```python
from build123d import *

# Parameters (mm, degrees)
F0_W        = 7.39
F0_H        = 23.34
F0_R        = 2.4
F1_DEPTH    = 7.88
F2_T1_DEPTH = 26.405
F4_DEPTH    = 7.391
F5_R        = 3.705


# Not quite as in the source:
# - a fillet or chamfer that OpenCascade refuses, or shapes differently, is made with other operations: its cross-section is extruded or revolved along the edge and cut away or added


with BuildPart() as f1:
    # F0 (on Top) → F1 (new body)
    with BuildSketch(Plane.XY):
        with Locations((-61.1013304442, -8.6294944299)):
            Rectangle(F0_W, F0_H)
        with Locations((-61.1013304442, -8.6294944299)):
            Circle(F0_R, mode=Mode.SUBTRACT)
        with Locations((-61.1013304442, -0.6294944299)):
            Circle(F0_R, mode=Mode.SUBTRACT)
    extrude(amount=F1_DEPTH)

    # F2: fillet of radius 3.705 on 2 edges, made by hand

    # F2_s2 → F2_t1 (cut)
    with BuildSketch(Plane.XY.offset(-9.2625)):
        with BuildLine():
            ThreePointArc((-61.0913304442, 3.0405055701), (-63.7111610685, 1.9553361944), (-64.7963304442, -0.6644944299))
            Line((-64.7963304442, -0.6644944299), (-64.7963304442, 3.0405055701))
            Line((-64.7963304442, 3.0405055701), (-61.0913304442, 3.0405055701))
        make_face()
        with BuildLine():
            ThreePointArc((-61.1113304442, 3.0405055701), (-58.4914998199, 1.9553361944), (-57.4063304442, -0.6644944299))
            Line((-57.4063304442, -0.6644944299), (-57.4063304442, 3.0405055701))
            Line((-57.4063304442, 3.0405055701), (-61.1113304442, 3.0405055701))
        make_face()
    extrude(amount=F2_T1_DEPTH, mode=Mode.SUBTRACT)

    # F3 (on face) → F4 (cut, through all)
    with BuildSketch(Plane.YZ.offset(-57.4063304442)):
        with BuildLine():
            Line((-15.7294944299, 5.34), (-15.7294944299, 6.0963858653))
            ThreePointArc((-15.7294944299, 6.0963858653), (-15.747402223, 6.1534898894), (-15.7947118212, 6.1901417725))
            ThreePointArc((-15.7947118212, 6.1901417725), (-16.6294944299, 6.34), (-17.4642770386, 6.1901417725))
            ThreePointArc((-17.4642770386, 6.1901417725), (-17.5115866368, 6.1534898894), (-17.5294944299, 6.0963858653))
            Line((-17.5294944299, 6.0963858653), (-17.5294944299, 5.34))
            ThreePointArc((-17.5294944299, 5.34), (-17.6759410393, 4.9864466094), (-18.0294944299, 4.84))
            Line((-18.0294944299, 4.84), (-18.7858802952, 4.84))
            ThreePointArc((-18.7858802952, 4.84), (-18.8429843193, 4.8220922069), (-18.8796362024, 4.7747826087))
            ThreePointArc((-18.8796362024, 4.7747826087), (-18.9917328021, 4.3640635248), (-19.0294944299, 3.94))
            ThreePointArc((-19.0294944299, 3.94), (-18.9917328021, 3.5159364752), (-18.8796362024, 3.1052173913))
            ThreePointArc((-18.8796362024, 3.1052173913), (-18.8429843193, 3.0579077931), (-18.7858802952, 3.04))
            Line((-18.7858802952, 3.04), (-18.0294944299, 3.04))
            ThreePointArc((-18.0294944299, 3.04), (-17.6759410393, 2.8935533906), (-17.5294944299, 2.54))
            Line((-17.5294944299, 2.54), (-17.5294944299, 1.7836141347))
            ThreePointArc((-17.5294944299, 1.7836141347), (-17.5115866368, 1.7265101106), (-17.4642770386, 1.6898582275))
            ThreePointArc((-17.4642770386, 1.6898582275), (-16.6294944299, 1.54), (-15.7947118212, 1.6898582275))
            ThreePointArc((-15.7947118212, 1.6898582275), (-15.747402223, 1.7265101106), (-15.7294944299, 1.7836141347))
            Line((-15.7294944299, 1.7836141347), (-15.7294944299, 2.54))
            ThreePointArc((-15.7294944299, 2.54), (-15.5830478205, 2.8935533906), (-15.2294944299, 3.04))
            Line((-15.2294944299, 3.04), (-14.4731085646, 3.04))
            ThreePointArc((-14.4731085646, 3.04), (-14.4160045405, 3.0579077931), (-14.3793526574, 3.1052173913))
            ThreePointArc((-14.3793526574, 3.1052173913), (-14.2672560577, 3.5159364752), (-14.2294944299, 3.94))
            ThreePointArc((-14.2294944299, 3.94), (-14.2672560577, 4.3640635248), (-14.3793526574, 4.7747826087))
            ThreePointArc((-14.3793526574, 4.7747826087), (-14.4160045405, 4.8220922069), (-14.4731085646, 4.84))
            Line((-14.4731085646, 4.84), (-15.2294944299, 4.84))
            ThreePointArc((-15.2294944299, 4.84), (-15.5830478205, 4.9864466094), (-15.7294944299, 5.34))
        make_face()
    extrude(amount=-F4_DEPTH, mode=Mode.SUBTRACT)

    # F5
    f5_edges = [f1.edges().sort_by_distance(p)[0] for p in [
        (-61.10133, -20.299494, 7.88),
        (-61.10133, -20.299494, 0),
    ]]
    fillet(f5_edges, radius=F5_R)


solid = f1.part
```
The model under review builds one solid part; all positions refer to its coordinate system, in mm. A direction names the side the tool comes from. Round coordinates to 2 decimals unless told otherwise and drop trailing zeros. Write each loop counter-clockwise with the first axis right and the second up, starting at its lowest first coordinate (ties: lowest second). Pieces come first, ordered by that corner, then holes. Notation, with made-up numbers: (-32, -21.5) - (-8, -21.5) arc R26 cw to (-8, 8.5) - close; hole circle Ø1 at (15.5, 61.25). An arc over 180 degrees is marked (long way). One line per question, with ' | ' between items.
Item 1: Add section B-B, the plane x = -62.25. State how many separate pieces and enclosed holes the cut face has, then the cut area to 3 significant figures.
Resolved:
separate pieces: 3 | enclosed holes: 1 | area: 96.3 mm2
Item 2: The part is to be moulded in two halves that separate along Y. For faces 1 (the face through (-63.686, 1.98, 3.885)), 2 (the face through (-59.5, -6.6, 0)), 3 (the face through (-59.994, -10.759, 3.885)), say which applies: pulls with the +Y half, pulls with the -Y half, needs draft (parallel to the pull), parting line crosses it, or undercut.
Resolved:
face 1: pulls with the +Y half | face 2: needs draft | face 3: undercut
Item 3: To check wall thickness, follow probe 1 along Y at (x, z) = (-62.5, 5); probe 2 along Y at (x, z) = (-61.75, 2); probe 3 along X at (y, z) = (-8.5, 2). State the ranges of each line that lie inside material, in increasing order.
Resolved:
probe 1: y = -20.21 to -17.66, -15.6 to -10.58, -6.68 to -2.58, 1.32 to 2.76 | probe 2: y = -19.88 to -17.53, -15.73 to -10.94, -6.32 to -2.94, 1.68 to 2.98 | probe 3: x = -64.8 to -63.5, -58.7 to -57.41
Item 4: For faces 4 (the face through (-61.05, -16.62, 6.34)), 5 (the face through (-59.5, -6.6, 7.88)), list the 3-axis set-ups (+Z, -Z, +X, -X, +Y, -Y) from which the entire face can be reached by the end or side of a thin tool; tool diameter is ignored.
Resolved:
face 4: +X, -X | face 5: +Z, +X, -X, +Y, -Y
Item 5: Add section A-A, the plane y = -14.75. Give the boundary of the cut face in (x, z), then the cut area to 3 significant figures.
Resolved:
outline: (-64.8, 0) - (-57.41, 0) - (-57.41, 3.04) - (-64.8, 3.04) - close; (-64.8, 4.84) - (-57.41, 4.84) - (-57.41, 7.88) - (-64.8, 7.88) - close | area: 44.9 mm2
Item 6: Add section C-C, the plane y = -10.75. Give the boundary of the cut face in (x, z).
Resolved:
outline: (-64.8, 0) - (-62.23, 0) - (-62.23, 7.88) - (-64.8, 7.88) - close; (-59.98, 0) - (-57.41, 0) - (-57.41, 7.88) - (-59.98, 7.88) - close
Item 7: For P1, Ø0.6, axis at x = -60.5, z = 5.5, coming from the +Y side; P2, Ø0.6, axis at x = -59.5, z = 2, coming from the +Y side; P3, Ø0.6, axis at x = -60, y = -18, coming from the +Z side, all flat-tipped, find the tip position at first contact; note any pin that passes through.
Resolved:
P1: stops at y = 3.03 | P2: stops at y = 2.8 | P3: stops at z = 7.71
